Design review of the part built by this model. Coordinates are the model's own, in mm. A direction names the side the tool comes from. Round coordinates to 2 decimals unless told otherwise and drop trailing zeros. Use CSV: the item, a comma, the result in double quotes.
from build123d import *

# Parameters (mm, degrees)
F1_DEPTH    = 3
F2_T1_DEPTH = 52.6928029293
F2_T4_ANGLE = 359.64
F2_T6_ANGLE = 359.64
F3_R        = 0.5


# Not quite as in the source:
# - a fillet or chamfer that OpenCascade refuses, or shapes differently, is made with other operations: its cross-section is extruded or revolved along the edge and cut away or added


with BuildPart() as f1:
    # F0 (on Top) → F1 (new body)
    with BuildSketch(Plane.XY):
        with BuildLine():
            Line((0, -21.2030354887), (0, 0))
            Line((0, 0), (-18.5486488044, 0))
            Line((-18.5486488044, 0), (-18.5486488044, -4.6107494656))
            Line((-18.5486488044, -4.6107494656), (-10.5158546939, -3.2809847035))
            ThreePointArc((-10.5158546939, -3.2809847035), (-8.3883004552, -5.7297930738), (-10.4765901342, -8.212170098))
            Line((-10.4765901342, -8.212170098), (-18.5486488044, -9.5484347937))
            Line((-18.5486488044, -9.5484347937), (-18.5486488044, -21.2030354887))
            Line((-18.5486488044, -21.2030354887), (0, -21.2030354887))
        make_face()
        with BuildLine():
            Line((-18.5486488044, -4.6107494656), (-18.5486488044, 0))
            Line((-18.5486488044, 0), (-132.8552216291, 0))
            ThreePointArc((-132.8552216291, 0), (-136.5013867617, -4.4477159734), (-140.1475518942, 0))
            Line((-140.1475518942, 0), (-152.0042717457, 0))
            Line((-152.0042717457, 0), (-152.0042717457, -42.4060709774))
            Line((-152.0042717457, -42.4060709774), (0, -42.4060709774))
            Line((0, -42.4060709774), (0, -21.2030354887))
            Line((0, -21.2030354887), (-18.5486488044, -21.2030354887))
            Line((-18.5486488044, -21.2030354887), (-18.5486488044, -9.5484347937))
            Line((-18.5486488044, -9.5484347937), (-118.7394559383, -26.1342208833))
            ThreePointArc((-118.7394559383, -26.1342208833), (-120.8670101771, -23.6854125129), (-118.7787204981, -21.2030354887))
            Line((-118.7787204981, -21.2030354887), (-18.5486488044, -4.6107494656))
        make_face()
    extrude(amount=F1_DEPTH)

    # F2: chamfer of 2 on 4 edges, made by hand

    # F2_s2 → F2_t1 (cut)
    with BuildSketch(Plane.XZ.offset(-5.1433659759)):
        Polygon((0, 1), (-2, 3), (0, 3), align=None)
        Polygon((0, 2), (-2, 0), (0, 0), align=None)
    extrude(amount=F2_T1_DEPTH, mode=Mode.SUBTRACT)

    # F2_s3 → F2_t4 (revolve, cut)
    with BuildSketch(Plane(origin=(-136.4977483257, 0.4288217341, 0), x_dir=(0, 0, 1), z_dir=(-0.9999950652, 0.0031415875, 0))):
        Polygon((1, 2.5602393555), (3, 4.5602393555), (3, 2.5602393555), align=None)
    revolve(axis=Axis((-136.5013867617, -0.7293245843, 3), (0, 0, -1)), revolution_arc=F2_T4_ANGLE, mode=Mode.SUBTRACT)

    # F2_s5 → F2_t6 (revolve, cut)
    with BuildSketch(Plane(origin=(-136.4977483257, 0.4288217341, 0), x_dir=(0, 0, 1), z_dir=(-0.9999950652, 0.0031415875, 0))):
        Polygon((2, 2.5602393555), (0, 4.5602393555), (0, 2.5602393555), align=None)
    revolve(axis=Axis((-136.5013867617, -0.7293245843, 0), (0, 0, -1)), revolution_arc=F2_T6_ANGLE, mode=Mode.SUBTRACT)

    # F3
    f3_edges = [f1.edges().sort_by_distance(p)[0] for p in [
        (-64.647288, -12.24201, 3),
        (-64.608023, -17.173195, 3),
        (-120.86701, -23.685413, 3),
        (-8.3883, -5.729793, 3),
        (-64.647288, -12.24201, 0),
        (-8.3883, -5.729793, 0),
        (-120.86701, -23.685413, 0),
    ]]
    fillet(f3_edges, radius=F3_R)


solid = f1.part
1) The part is to be moulded in two halves that separate along X. For faces 4 (the face through (-78, -21, 0)), 5 (the face through (-136.392, -5.207, 1.76)), 6 (the face through (-152.004, -21, 1)), say which applies: +X half, -X half, draft (parallel to the pull), parting line (faces both ways), or undercut.
Data:
face 4,"draft"
face 5,"undercut"
face 6,"-X half"
2) For faces 1 (the face through (-65.379, -17.453, 0.143)), 2 (the face through (-63.85, -17.048, 1.486)), 3 (the face through (-65.379, -17.453, 2.857)), list the 3-axis set-ups (+Z, -Z, +X, -X, +Y, -Y) from which the entire face can be reached by the end or side of a thin tool; tool diameter is ignored.
Data:
face 1,"-Z"
face 2,"+Z, -Z"
face 3,"+Z"
3) To check wall thickness, follow L1, parallel to Y at x = -34.5, z = 1.85; L2, parallel to Y at x = -107.5, z = 2; L3, parallel to X at y = -1.5, z = 0.8. State the ranges of each line that lie inside material, in increasing order. Write a range as from..to.
Data:
L1,"y = -42.41..-12.19, -7.25..0"
L2,"y = -42.41..-24.27, -19.34..0"
L3,"x = -152..-141.36, -131.64..-1.2"
4) Insertion check: pin 1 Ø4 at (x, y) = (-73, -36) entering from -Z. The pin has a flat end and moves straight along its axis. Give the tip position at first contact, or say it passes through.
Data:
pin 1,"stops at z = 0"
